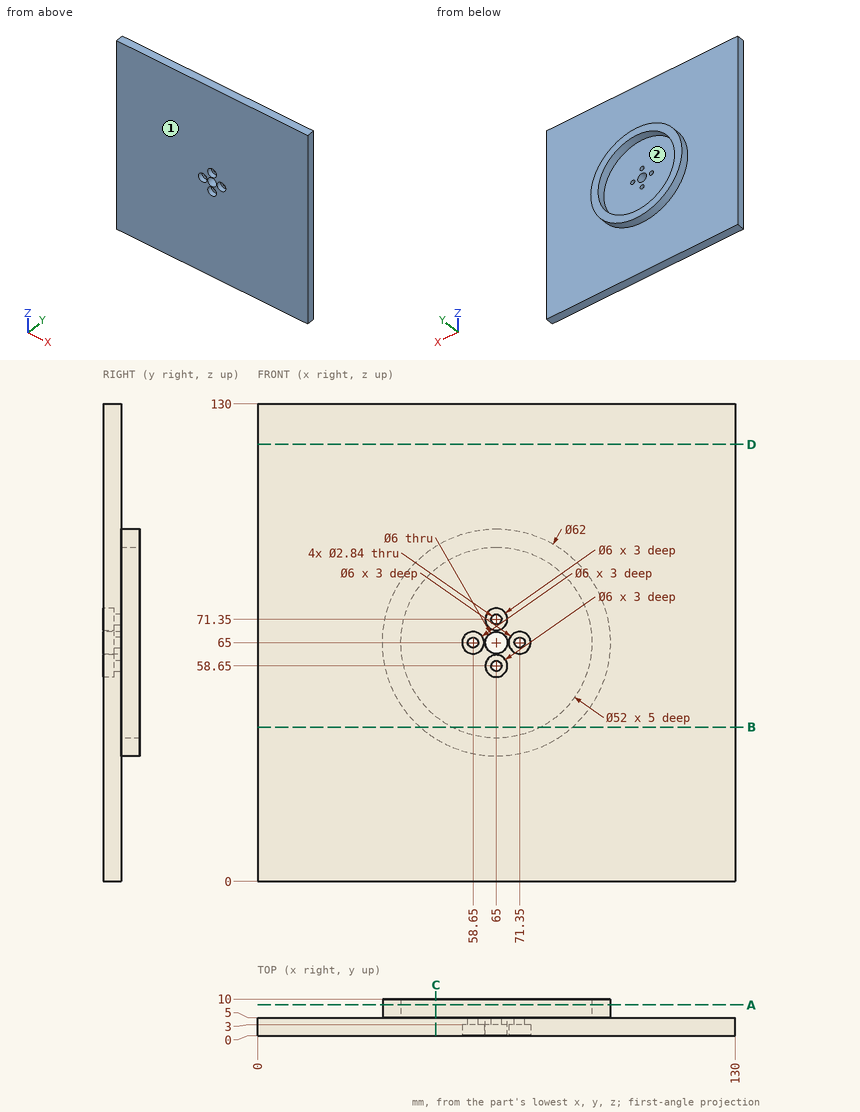
Drawing for the job (mm, zero at the part's lowest x, y, z). Round coordinates to 2 decimals unless told otherwise and drop trailing zeros. Write each loop counter-clockwise with the first axis right and the second up, starting at its lowest first coordinate (ties: lowest second). Pieces come first, ordered by that corner, then holes. Notation, with made-up numbers: (72, -40) - (91, -40) arc R25 ccw to (91, -10) - close; hole circle Ø10 at (-24.75, -7). An arc over 180 degrees is marked (long way). Write item = value, one per line. Start each with the question number.
Q1. Band-saw the part on B-B (z = 42). Give the cut face in (x, y).
Q2. Probe L1, parallel to X at y = 1.85, z = 65; L2, parallel to Y at x = 72, z = 14; L3, parallel to X at y = 1.6, z = 71.35. List the from-to ranges inside material, lowest first. Write a range as from..to.
Q3. Band-saw the part on A-A (y = 8.5). Give the cut face in (x, z).
Q4. Drop flat-ended pins along their axis: pin 1 (3.5 mm diameter, centred on x = 71.35, z = 65, fed in from -Y); pin 2 (8 mm diameter, centred on x = 58.65, z = 65, fed in from -Y); pin 3 (4 mm diameter, centred on x = 99, z = 109, fed in from +Y); pin 4 (2 mm diameter, centred on y = 8, z = 75, fed in from +X). Give the stop position or say it passes through.
Q5. Band-saw the part on D-D (z = 119). Give the cut face in (x, y), then the cut area to 3 significant figures.
Q6. Band-saw the part on C-C (x = 48.5). Give the cut face in (y, z), then the cut area to 3 significant figures.
Q7. Mould opens along Z. For the marked faces 1 and 2 say: pulls with the +Z half, pulls with the -Z half, needs draft (parallel to the pull), parting line crosses it, or undercut.
Answers below:
q1.outline = (0, 0) - (130, 0) - (130, 5) - (85.78, 5) - (85.78, 10) - (77.12, 10) - (77.12, 5) - (52.88, 5) - (52.88, 10) - (44.22, 10) - (44.22, 5) - (0, 5) - close
q2.L1 = 0..55.65, 61.65..62, 68..68.35, 74.35..130
q2.L2 = 0..5
q2.L3 = 0..62, 68..130
q3.outline = circle Ø62 at (65, 65); hole circle Ø52 at (65, 65)
q4.pin_1 = 3
q4.pin_2 = 0
q4.pin_3 = 5
q4.pin_4 = 94.66
q5.outline = (0, 0) - (130, 0) - (130, 5) - (0, 5) - close
q5.area = 650 mm2
q6.outline = (0, 0) - (5, 0) - (5, 38.76) - (10, 38.76) - (10, 44.91) - (5, 44.91) - (5, 85.09) - (10, 85.09) - (10, 91.24) - (5, 91.24) - (5, 130) - (0, 130) - close
q6.area = 712 mm2
q7.face_1 = needs draft
q7.face_2 = undercut
